The listing builds one solid part. Answer for the finished solid, in the listing's coordinates (mm). Face numbers are marked on the shaded views. A direction names the side the tool comes from. Give positions to 0.01 mm unless a question says otherwise; leave off trailing zeros. Loops run counter-clockwise (first coordinate to the right, second up) from the corner with the lowest first, then second, coordinate; pieces in that order, holes last. Notation, with made-up numbers: (19, 76) - (61, 76) arc R16 cw to (61, 102) - close; hole circle Ø10 at (37.5, 63). An arc over 180 degrees is marked (long way). Answer as CSV lines item,"result". Start each with the question number.
1) A cutting plane is placed at C-C (z = 3). Give the number of separate pieces and of enclosed holes in the cut face, and give its area (3 significant figures).
2) A cutting plane is placed at A-A (y = 5.5). Determine the outline of the cut face in (x, z).
3) Find the intervals of material crossed by line 1 along X through (y, z) = (-25.5, 1.5); line 2 along Y through (x, z) = (38.55, 3); line 3 along X through (y, z) = (0, 4), in increasing order.
4) For a pull along X with two mould halves and no side action, classify the marked faces 1 and 2 as pulls with the +X half, pulls with the -X half, needs draft (parallel to the pull), parting line crosses it, or undercut.
5) For the marked faces 3 and 4, determine the directions among +Z, -Z, +X, -X, +Y, -Y from which every point of the face is accessible in a straight line to the end or side of a thin tool.
6) Flat-ended cylindrical pins translate along their axes: pin 1 (0.9 mm diameter, centred on y = 0, z = 2.5, fed in from +X); pin 2 (10 mm diameter, centred on x = 8, y = 18.5, fed in from +Z). Find the tip coordinate at first contact, or state that the pin passes through.
7) A cutting plane is placed at B-B (x = -16). Determine the outline of the cut face in (y, z), and give its area (3 significant figures).
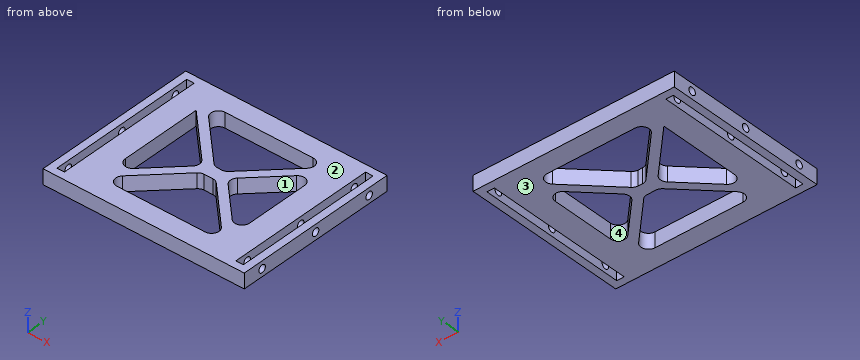
```python
from build123d import *

# Parameters (mm, degrees)
SKETCH1_W           = 81
SKETCH1_H           = 66
BOSS_EXTRUDE1_DEPTH = 6
SKETCH3_W           = 3
SKETCH3_H           = 60
CUT_EXTRUDE2_DEPTH  = 7
CUT_EXTRUDE5_DEPTH  = 7
FILLET2_R           = 3
FILLET3_R           = 3
SKETCH6_R           = 1.5
CUT_EXTRUDE6_DEPTH  = 10


with BuildPart() as part:
    # Sketch1 → Boss-Extrude1 (new body)
    with BuildSketch(Plane.XY):
        Rectangle(SKETCH1_W, SKETCH1_H)
    extrude(amount=BOSS_EXTRUDE1_DEPTH)

    # Sketch3 → Cut-Extrude2 (cut, through all)
    with BuildSketch(Plane.XY.offset(6)):
        with Locations((-36, 0)):
            Rectangle(SKETCH3_W, SKETCH3_H)
        with Locations((36, 0)):
            Rectangle(SKETCH3_W, SKETCH3_H)
    extrude(amount=-CUT_EXTRUDE2_DEPTH, mode=Mode.SUBTRACT)

    # Sketch5 → Cut-Extrude5 (cut, through all)
    with BuildSketch(Plane.XY.offset(6)):
        Polygon((-5, 0), (-25, 20), (-25, -20), align=None)
        Polygon((-3, -3), (-25, -25), (0, -25), (0, -3), align=None)
        Polygon((0, -3), (0, -25), (25, -25), (3, -3), align=None)
        Polygon((25, -20), (25, 20), (5, 0), align=None)
        Polygon((25, 25), (0, 25), (0, 2.121320344), (2.121320344, 2.121320344), align=None)
        Polygon((0, 25), (-25, 25), (-2.121320344, 2.121320344), (0, 2.121320344), align=None)
    extrude(amount=-CUT_EXTRUDE5_DEPTH, mode=Mode.SUBTRACT)

    # Fillet2
    fillet2_edges = [part.edges().sort_by_distance(p)[0] for p in [
        (25, 20, 3),
        (25, -20, 3),
        (25, -25, 3),
        (-25, -25, 3),
        (-25, 25, 3),
        (25, 25, 3),
        (-25, -20, 3),
    ]]
    fillet(fillet2_edges, radius=FILLET2_R)

    # Fillet3
    fillet3_edges = [part.edges().sort_by_distance(p)[0] for p in [
        (5, 0, 3),
        (-3, -3, 3),
        (3, -3, 3),
        (2.121320344, 2.121320344, 3),
        (-2.121320344, 2.121320344, 3),
        (-5, 0, 3),
    ]]
    fillet(fillet3_edges, radius=FILLET3_R)

    # Sketch6 → Cut-Extrude6 (cut)
    with BuildSketch(Plane.ZY.offset(40.5)):
        with Locations((3, 24.75)):
            Circle(SKETCH6_R)
        with Locations((3, 0)):
            Circle(SKETCH6_R)
        with Locations((3, -24.75)):
            Circle(SKETCH6_R)
    cut_extrude6 = extrude(amount=-CUT_EXTRUDE6_DEPTH, mode=Mode.SUBTRACT)

    # Mirror1: Cut-Extrude6 across plane
    add(cut_extrude6.mirror(Plane(origin=(0, 0, 0), x_dir=(0, 0, 1), z_dir=(1, 0, 0))), mode=Mode.SUBTRACT)


solid = part.part
```
Ans:
1,separate pieces,"5"
1,enclosed holes,"4"
1,area,"2,910 mm2"
2,outline,"(-40.5, 0) - (-37.5, 0) - (-37.5, 6) - (-40.5, 6) - close; (-34.5, 0) - (-25, 0) - (-25, 6) - (-34.5, 6) - close; (-10.5, 0) - (-5.5, 0) - (-5.5, 6) - (-10.5, 6) - close; (5.5, 0) - (10.5, 0) - (10.5, 6) - (5.5, 6) - close; (25, 0) - (34.5, 0) - (34.5, 6) - (25, 6) - close; (37.5, 0) - (40.5, 0) - (40.5, 6) - (37.5, 6) - close"
3,line 1,"-40.5 to -37.5, -34.5 to 34.5, 37.5 to 40.5"
3,line 2,"-33 to -26.25, -23.25 to -1.5, 1.5 to 23.25, 26.25 to 33"
3,line 3,"-30.5 to -25, -6.24 to 6.24, 25 to 30.5"
4,face 1,"undercut"
4,face 2,"needs draft"
5,face 3,"-Z, +X, -X, +Y, -Y"
5,face 4,"+Z, -Z"
6,pin 1,"x = 30.5"
6,pin 2,"through"
7,outline,"(-33, 0) - (-25, 0) - (-25, 6) - (-33, 6) - close; (-16, 0) - (-11, 0) - (-11, 6) - (-16, 6) - close; (11, 0) - (16, 0) - (16, 6) - (11, 6) - close; (25, 0) - (33, 0) - (33, 6) - (25, 6) - close"
7,area,"156 mm2"
